Could you check a few things on this model? Use its own coordinates, in mm. Coordinates: 2 decimals unless noted, no trailing zeros. Loops run counter-clockwise (first coordinate to the right, second up) from the corner with the lowest first, then second, coordinate; pieces in that order, holes last.
1) Will this pin go through, and if not, where does the flat tip stop? P1, Ø4.5, axis at x = -48.5, z = 11.5, coming from the -Y side.
2) If I drill on line 1 along X through (y, z) = (-0.1, -11.5); line 2 along Z through (x, y) = (48.5, -0.05); line 3 along Z through (x, y) = (47, -1.1), over which ranges is the centre line in solid material (lowest first)?
3) Imagine slicing it at A-A on y = -0.9. Please give me the cut outline in (x, z), plus the area to 3 significant figures.
```python
from build123d import *

# Parameters (mm, degrees)
SKETCH_W         = 104.8
SKETCH_H         = 31
PAD_DEPTH        = 1.5
HOLE_D           = 3.4
HOLE_DEPTH       = 25
HOLE_CSINK_D     = 6.1
HOLE_CSINK_ANGLE = 90
FILLET_R         = 3.5


with BuildPart() as part:
    # Sketch → Pad (new body)
    with BuildSketch(Plane.XZ):
        Rectangle(SKETCH_W, SKETCH_H)
    extrude(amount=PAD_DEPTH)

    # Hole
    with Locations(Plane.XZ.offset(1.5)):
        with Locations((-48.5, 11.5), (-48.5, -11.5), (48.5, -11.5), (48.5, 11.5)):
            CounterSinkHole(HOLE_D / 2, HOLE_CSINK_D / 2, depth=HOLE_DEPTH, counter_sink_angle=HOLE_CSINK_ANGLE)

    # Fillet
    fillet_edges = [part.edges().sort_by_distance(p)[0] for p in [
        (-52.4, -0.75, 15.5),
        (52.4, -0.75, 15.5),
    ]]
    fillet(fillet_edges, radius=FILLET_R)


solid = part.part
```
Filled in:
1. P1: stops at y = -0.7
2. line 1: x = -52.4 to -50.2, -46.8 to 46.8, 50.2 to 52.4
2. line 2: z = -15.5 to -13.2, -9.8 to 9.8, 13.2 to 15.5
2. line 3: z = -15.5 to -13.68, -9.32 to 9.32, 13.68 to 15.5
3. outline: (-52.4, -15.5) - (52.4, -15.5) - (52.4, 12) arc R3.5 ccw to (48.9, 15.5) - (-48.9, 15.5) arc R3.5 ccw to (-52.4, 12) - close; hole circle Ø4.9 at (-48.5, -11.5); hole circle Ø4.9 at (-48.5, 11.5); hole circle Ø4.9 at (48.5, -11.5); hole circle Ø4.9 at (48.5, 11.5)
3. area: 3,170 mm2
